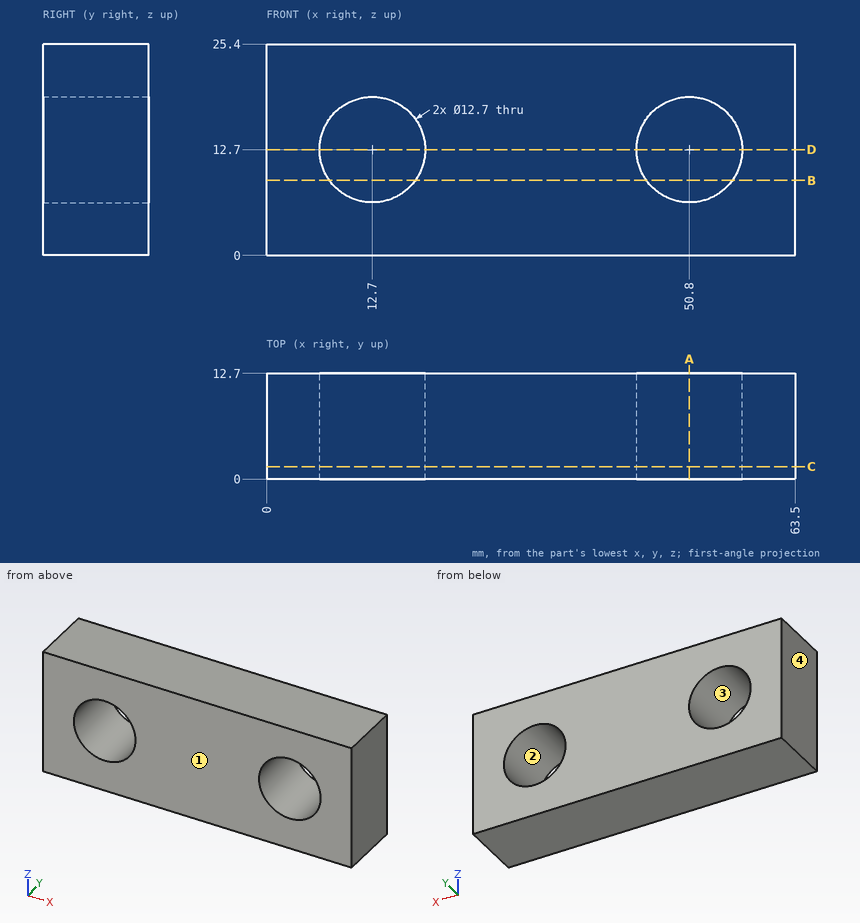
Input: dimensioned drawing with shaded views. Units: mm. Origin: part minimum x, y, z. Give positions to 0.01 mm unless a question says otherwise; leave off trailing zeros. Write each loop counter-clockwise with the first axis right and the second up, starting at its lowest first coordinate (ties: lowest second). Pieces come first, ordered by that corner, then holes.
1. Section query C-C (y = 1.5). Return the cut outline in (x, z).
2. First-contact query: pin 1 (5 mm diameter, centred on y = 9.5, z = 8, fed in from -X). Flat tip, straight axial feed; report the tip coordinate or a pass-through.
3. Material intervals for line 1 along X through (y, z) = (2.75, 12.75); line 2 along Z through (x, y) = (50.8, 5.5); line 3 along X through (y, z) = (2.75, 14.75), sorted ascending.
4. Section query B-B (z = 9). Return the cut outline in (x, y), then the cut area to 3 significant figures.
5. Section query A-A (x = 50.8). Return the cut outline in (y, z), then the cut area to 3 significant figures.
6. Section query D-D (z = 12.7). Return the cut outline in (x, y).
7. Pull-direction query (X, two-part tool) for the marked faces 1, 2, 3 and 4; classes: +X half, -X half, draft (parallel to the pull), parting line (faces both ways), or undercut.
Output values:
1. outline: (0, 0) - (63.5, 0) - (63.5, 25.4) - (0, 25.4) - close; hole circle Ø12.7 at (12.7, 12.7); hole circle Ø12.7 at (50.8, 12.7)
2. pin 1: stops at x = 0
3. line 1: x = 0 to 6.35, 19.05 to 44.45, 57.15 to 63.5
3. line 2: z = 0 to 6.35, 19.05 to 25.4
3. line 3: x = 0 to 6.69, 18.71 to 44.79, 56.81 to 63.5
4. outline: (0, 0) - (7.54, 0) - (7.54, 12.7) - (0, 12.7) - close; (17.86, 0) - (45.64, 0) - (45.64, 12.7) - (17.86, 12.7) - close; (55.96, 0) - (63.5, 0) - (63.5, 12.7) - (55.96, 12.7) - close
4. area: 544 mm2
5. outline: (0, 0) - (12.7, 0) - (12.7, 6.35) - (0, 6.35) - close; (0, 19.05) - (12.7, 19.05) - (12.7, 25.4) - (0, 25.4) - close
5. area: 161 mm2
6. outline: (0, 0) - (6.35, 0) - (6.35, 12.7) - (0, 12.7) - close; (19.05, 0) - (44.45, 0) - (44.45, 12.7) - (19.05, 12.7) - close; (57.15, 0) - (63.5, 0) - (63.5, 12.7) - (57.15, 12.7) - close
7. face 1: draft
7. face 2: undercut
7. face 3: undercut
7. face 4: -X half
